```python
from build123d import *

# Parameters (mm, degrees)
F0_W     = 1066.8
F0_H     = 76.2
F1_DEPTH = 44.45
F2_W     = 990.6
F2_H     = 19.05
F3_DEPTH = 50.8
F4_W     = 12.7
F4_H     = 12.7
F5_DEPTH = 44.451


with BuildPart() as f1:
    # F0 (on Top) → F1 (new body)
    with BuildSketch(Plane.XY):
        with Locations((406.253795, -0.947985)):
            Rectangle(F0_W, F0_H)
    extrude(amount=F1_DEPTH)

    # F2 (on face) → F3 (cut)
    with BuildSketch(Plane(origin=(0, 37.152015, 0), x_dir=(-1, 0, 0), z_dir=(0, 1, 0))):
        with Locations((-406.253795, 22.225)):
            Rectangle(F2_W, F2_H)
    extrude(amount=-F3_DEPTH, mode=Mode.SUBTRACT)

    # F4 (on face) → F5 (cut, through all)
    with BuildSketch(Plane(origin=(0, 0, 0), x_dir=(1, 0, 0), z_dir=(0, 0, -1))):
        with Locations((-31.896205, -11.752015)):
            Rectangle(F4_W, F4_H)
        with Locations((91.928795, -11.752015)):
            Rectangle(F4_W, F4_H)
        with Locations((244.328795, -11.752015)):
            Rectangle(F4_W, F4_H)
        with Locations((406.253795, -11.752015)):
            Rectangle(F4_W, F4_H)
        with Locations((568.178795, -11.752015)):
            Rectangle(F4_W, F4_H)
        with Locations((720.578795, -11.752015)):
            Rectangle(F4_W, F4_H)
        with Locations((844.403795, -11.752015)):
            Rectangle(F4_W, F4_H)
    extrude(amount=-F5_DEPTH, mode=Mode.SUBTRACT)


solid = f1.part
```
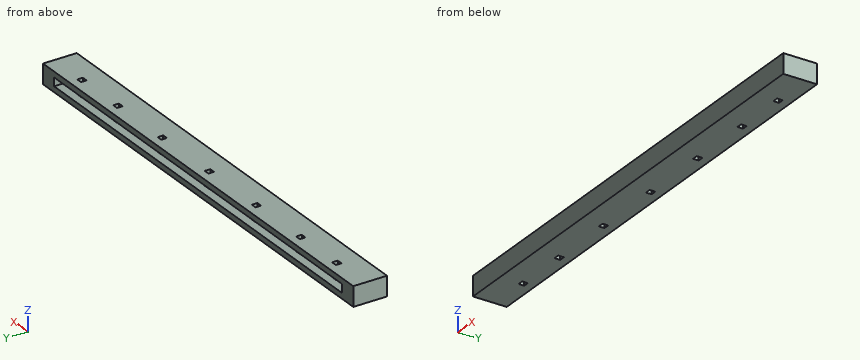
Input: part model. Units: mm. Frame: model coordinates. Give positions to 0.01 mm unless a question says otherwise; leave off trailing zeros. Order: outer loops, then holes, each group sorted by start corner. A loop starts at its lowest first (then second) coordinate and runs counter-clockwise, first axis right, second up.
1. Pin query (flat end, axial travel): pin 1 Ø1 at (x, y) = (376.5, 19) entering from -Z. Return the tip coordinate at first contact, or that it passes through.
Computed:
pin 1: stops at z = 0
2. Line query: probe 1 along X at (y, z) = (23.5, 29); probe 2 along Z at (x, y) = (125, 25); probe 3 along Y at (x, z) = (400, 34.5). Output: solid intervals per line, ascending.
Computed:
probe 1: x = -127.15 to -89.05, 901.55 to 939.65
probe 2: z = 0 to 12.7, 31.75 to 44.45
probe 3: y = -39.05 to 5.4, 18.1 to 37.15
3. Cut plane A-A (y = 28). Return loops of the section in (x, z).
Computed:
outline: (-127.15, 0) - (939.65, 0) - (939.65, 44.45) - (-127.15, 44.45) - close; hole (-89.05, 12.7) - (901.55, 12.7) - (901.55, 31.75) - (-89.05, 31.75) - close
4. Cut plane C-C (x = 286). Return loops of the section in (y, z).
Computed:
outline: (-39.05, 0) - (37.15, 0) - (37.15, 12.7) - (-13.65, 12.7) - (-13.65, 31.75) - (37.15, 31.75) - (37.15, 44.45) - (-39.05, 44.45) - close
5. Cut plane B-B (z = 20). Return loops of the section in (x, y).
Computed:
outline: (-127.15, -39.05) - (939.65, -39.05) - (939.65, 37.15) - (901.55, 37.15) - (901.55, -13.65) - (-89.05, -13.65) - (-89.05, 37.15) - (-127.15, 37.15) - close
